from build123d import *

# Parameters (mm, degrees)
EXTRUSION1_DEPTH        = 5
ESQUISSE3_R             = 1.5
ENL_V_MAT_EXTRU_1_DEPTH = 30.086079144
TROU_TARAUD_M3X0_51_D   = 2.5


with BuildPart() as part:
    # Esquisse1 → Extrusion1 (new body)
    with BuildSketch(Plane.XY):
        Polygon((-25, 0), (-17, 0), (-17, 4), (17, 4), (17, 0), (25, 0), (25, 14), (-25, 14), align=None)
    extrude(amount=EXTRUSION1_DEPTH)

    # Esquisse3 → Enlèv. mat.-Extru.1 (cut, through all)
    with BuildSketch(Plane(origin=(0, 14, 0), x_dir=(1, 0, 0), z_dir=(0, 1, 0))):
        with Locations(Location((13, -2.5, 0), (0, 0, 270))):
            Circle(ESQUISSE3_R)
        with Locations(Location((-13, -2.5, 0), (0, 0, 270))):
            Circle(ESQUISSE3_R)
    extrude(amount=-ENL_V_MAT_EXTRU_1_DEPTH, mode=Mode.SUBTRACT)

    # Trou taraudé M3x0.51 (through all)
    with Locations(Plane.XZ):
        with Locations((-21, 2.5), (21, 2.5)):
            Hole(TROU_TARAUD_M3X0_51_D / 2)


solid = part.part
Can you work these out from the model? Positions are in its coordinate system, mm. A direction names the side the tool comes from. Coordinates: 2 decimals unless noted, no trailing zeros. Order: outer loops, then holes, each group sorted by start corner. A loop starts at its lowest first (then second) coordinate and runs counter-clockwise, first axis right, second up. Notation, with made-up numbers: (8, 86) - (48, 86) arc R20 cw to (48, 106) - close; hole circle Ø2 at (39.5, 72). An arc over 180 degrees is marked (long way). Answer as a JSON object with one key per item and string values. Group by question number.
Q1. I need wall thicknesses on line 1 (Z direction, x = 21, y = 9); line 2 (X direction, y = 6, z = 2.2); line 3 (X direction, y = 10.5, z = 3.15). Which ranges of each line are inside material? Lowest first, please. Write a range as from..to.
Q2. Imagine slicing it at B-B (x = 21). Please give me the cut outline in (y, z).
Q3. We'd pull the mould along X, two halves only. Please class faces 1 (the face through (13, 9, 1)), 2 (the face through (-25, 7, 2)), 3 (the face through (0, 9, 5)): +X half, -X half, draft (parallel to the pull), parting line (faces both ways), or undercut.
Q4. Imagine slicing it at A-A (z = 2.5). Please give me the cut outline in (x, y).
Q5. Imagine slicing it at C-C (y = 10). Please give me the cut outline in (x, z).
Q6. Imagine slicing it at D-D (x = 13). Please give me the cut outline in (y, z), and give its area (3 significant figures).
Q7. On a 3-axis mill with a long thin cutter (end or side, diameter ignored), from which of +Z, -Z, +X, -X, +Y, -Y can I reach the whole of each face in a straight line? I mean faces 4 (the face through (19.845, 7.098, 2.021)), 5 (the face through (0, 4, 2)). Say none if no direction works.
Determined:
{
 "1": {"line 1": "z = 0..1.25, 3.75..5", "line 2": "x = -25..-22.21, -19.79..-14.47, -11.53..11.53, 14.47..19.79, 22.21..25", "line 3": "x = -25..-22.07, -19.93..-14.35, -11.65..11.65, 14.35..19.93, 22.07..25"},
 "2": {"outline": "(0, 0) - (14, 0) - (14, 1.25) - (0, 1.25) - close; (0, 3.75) - (14, 3.75) - (14, 5) - (0, 5) - close"},
 "3": {"face 1": "undercut", "face 2": "-X half", "face 3": "draft"},
 "4": {"outline": "(-25, 0) - (-22.25, 0) - (-22.25, 14) - (-25, 14) - close; (-19.75, 0) - (-17, 0) - (-17, 4) - (-14.5, 4) - (-14.5, 14) - (-19.75, 14) - close; (-11.5, 4) - (11.5, 4) - (11.5, 14) - (-11.5, 14) - close; (14.5, 4) - (17, 4) - (17, 0) - (19.75, 0) - (19.75, 14) - (14.5, 14) - close; (22.25, 0) - (25, 0) - (25, 14) - (22.25, 14) - close"},
 "5": {"outline": "(-25, 0) - (25, 0) - (25, 5) - (-25, 5) - close; hole circle Ø2.5 at (-21, 2.5); hole circle Ø3 at (-13, 2.5); hole circle Ø3 at (13, 2.5); hole circle Ø2.5 at (21, 2.5)"},
 "6": {"outline": "(4, 0) - (14, 0) - (14, 1) - (4, 1) - close; (4, 4) - (14, 4) - (14, 5) - (4, 5) - close", "area": "20.0 mm2"},
 "7": {"face 4": "+Y, -Y", "face 5": "+Z, -Z, -Y"}
}
